The listing builds one solid part. Answer for the finished solid, in the listing's coordinates (mm). Round coordinates to 2 decimals unless told otherwise and drop trailing zeros. Write each loop counter-clockwise with the first axis right and the second up, starting at its lowest first coordinate (ties: lowest second). Pieces come first, ordered by that corner, then holes. Notation, with made-up numbers: M -2,88 L 36,88 A25 cw 36,123 Z; hole C 64,78.25 d3. An arc over 180 degrees is marked long. Answer as CSV lines item,"result". Start each with the question number.
from build123d import *

# Parameters (mm, degrees)
SKETCH22_R                       = 2.15
F_20_SERIES_TS20_40B_5MM_1_DEPTH = 225
M6X1_0_TAPPED_HOLE2_D            = 5
M6X1_0_TAPPED_HOLE2_DEPTH        = 15
M6X1_0_TAPPED_HOLE2_TIP          = 1.502151548


with BuildPart() as part:
    # Sketch22 → 20 series TS20-40B_5MM(1) (new body)
    with BuildSketch(Plane(origin=(0, 0, 0), x_dir=(-1, 0, 0), z_dir=(0, 1, 0))):
        with BuildLine():
            Line((-9.5, 7), (-8.476, 7))
            Line((-8.476, 7), (-8.476, 4.05))
            Line((-8.476, 4.05), (-7.063551759, 4.05))
            Line((-7.063551759, 4.05), (-4.5, 6.613551759))
            Line((-4.5, 6.613551759), (-4.5, 13.386448241))
            Line((-4.5, 13.386448241), (-7.063551759, 15.95))
            Line((-7.063551759, 15.95), (-8.476, 15.95))
            Line((-8.476, 15.95), (-8.476, 13))
            Line((-8.476, 13), (-9.5, 13))
            Line((-9.5, 13), (-9.5, 13.5))
            Line((-9.5, 13.5), (-10, 13.5))
            Line((-10, 13.5), (-10, 18.5014))
            ThreePointArc((-10, 18.5014), (-9.561070222, 19.561070222), (-8.5014, 20))
            Line((-8.5014, 20), (-3.5, 20))
            Line((-3.5, 20), (-3.5, 19.5))
            Line((-3.5, 19.5), (-3, 19.5))
            Line((-3, 19.5), (-3, 18.476))
            Line((-3, 18.476), (-5.95, 18.476))
            Line((-5.95, 18.476), (-5.95, 17.063551759))
            Line((-5.95, 17.063551759), (-3.386448241, 14.5))
            Line((-3.386448241, 14.5), (3.386448241, 14.5))
            Line((3.386448241, 14.5), (5.95, 17.063551759))
            Line((5.95, 17.063551759), (5.95, 18.476))
            Line((5.95, 18.476), (3, 18.476))
            Line((3, 18.476), (3, 19.5))
            Line((3, 19.5), (3.5, 19.5))
            Line((3.5, 19.5), (3.5, 20))
            Line((3.5, 20), (8.5014, 20))
            ThreePointArc((8.5014, 20), (9.561070222, 19.561070222), (10, 18.5014))
            Line((10, 18.5014), (10, 13.5))
            Line((10, 13.5), (9.5, 13.5))
            Line((9.5, 13.5), (9.5, 13))
            Line((9.5, 13), (8.476, 13))
            Line((8.476, 13), (8.476, 15.95))
            Line((8.476, 15.95), (7.063551759, 15.95))
            Line((7.063551759, 15.95), (4.5, 13.386448241))
            Line((4.5, 13.386448241), (4.5, 6.613551759))
            Line((4.5, 6.613551759), (7.063551759, 4.05))
            Line((7.063551759, 4.05), (8.476, 4.05))
            Line((8.476, 4.05), (8.476, 7))
            Line((8.476, 7), (9.5, 7))
            Line((9.5, 7), (9.5, 6.5))
            Line((9.5, 6.5), (10, 6.5))
            Line((10, 6.5), (10, -6.5))
            Line((10, -6.5), (9.5, -6.5))
            Line((9.5, -6.5), (9.5, -7))
            Line((9.5, -7), (8.476, -7))
            Line((8.476, -7), (8.476, -4.05))
            Line((8.476, -4.05), (7.063551759, -4.05))
            Line((7.063551759, -4.05), (4.5, -6.613551759))
            Line((4.5, -6.613551759), (4.5, -13.386448241))
            Line((4.5, -13.386448241), (7.063551759, -15.95))
            Line((7.063551759, -15.95), (8.476, -15.95))
            Line((8.476, -15.95), (8.476, -13))
            Line((8.476, -13), (9.5, -13))
            Line((9.5, -13), (9.5, -13.5))
            Line((9.5, -13.5), (10, -13.5))
            Line((10, -13.5), (10, -18.5014))
            ThreePointArc((10, -18.5014), (9.561070222, -19.561070222), (8.5014, -20))
            Line((8.5014, -20), (3.5, -20))
            Line((3.5, -20), (3.5, -19.5))
            Line((3.5, -19.5), (3, -19.5))
            Line((3, -19.5), (3, -18.476))
            Line((3, -18.476), (5.95, -18.476))
            Line((5.95, -18.476), (5.95, -17.063551759))
            Line((5.95, -17.063551759), (3.386448241, -14.5))
            Line((3.386448241, -14.5), (-3.386448241, -14.5))
            Line((-3.386448241, -14.5), (-5.95, -17.063551759))
            Line((-5.95, -17.063551759), (-5.95, -18.476))
            Line((-5.95, -18.476), (-3, -18.476))
            Line((-3, -18.476), (-3, -19.5))
            Line((-3, -19.5), (-3.5, -19.5))
            Line((-3.5, -19.5), (-3.5, -20))
            Line((-3.5, -20), (-8.5014, -20))
            ThreePointArc((-8.5014, -20), (-9.561070222, -19.561070222), (-10, -18.5014))
            Line((-10, -18.5014), (-10, -13.5))
            Line((-10, -13.5), (-9.5, -13.5))
            Line((-9.5, -13.5), (-9.5, -13))
            Line((-9.5, -13), (-8.476, -13))
            Line((-8.476, -13), (-8.476, -15.95))
            Line((-8.476, -15.95), (-7.063551759, -15.95))
            Line((-7.063551759, -15.95), (-4.5, -13.386448241))
            Line((-4.5, -13.386448241), (-4.5, -6.613551759))
            Line((-4.5, -6.613551759), (-7.063551759, -4.05))
            Line((-7.063551759, -4.05), (-8.476, -4.05))
            Line((-8.476, -4.05), (-8.476, -7))
            Line((-8.476, -7), (-9.5, -7))
            Line((-9.5, -7), (-9.5, -6.5))
            Line((-9.5, -6.5), (-10, -6.5))
            Line((-10, -6.5), (-10, 6.5))
            Line((-10, 6.5), (-9.5, 6.5))
            Line((-9.5, 6.5), (-9.5, 7))
        make_face()
        with Locations((0, 10)):
            Circle(SKETCH22_R, mode=Mode.SUBTRACT)
        with Locations((0, -10)):
            Circle(SKETCH22_R, mode=Mode.SUBTRACT)
        Polygon((-3.45829029, 5.5), (-6.43229029, 2.526), (-8.476, 2.526), (-8.476, -2.526), (-6.43229029, -2.526), (-3.45829029, -5.5), (3.45829029, -5.5), (6.43229029, -2.526), (8.476, -2.526), (8.476, 2.526), (6.43229029, 2.526), (3.45829029, 5.5), align=None, mode=Mode.SUBTRACT)
    extrude(amount=F_20_SERIES_TS20_40B_5MM_1_DEPTH)

    # M6x1.0 Tapped Hole2
    with Locations(Plane(origin=(0, 0, 0), x_dir=(-1, 0, 0), z_dir=(0, -1, 0))):
        with Locations((0, 10), (0, -10)):
            Hole(M6X1_0_TAPPED_HOLE2_D / 2, depth=M6X1_0_TAPPED_HOLE2_DEPTH)
            with Locations((0, 0, -(M6X1_0_TAPPED_HOLE2_DEPTH + M6X1_0_TAPPED_HOLE2_TIP / 2))):  # 118° drill point
                Cone(0, M6X1_0_TAPPED_HOLE2_D / 2, M6X1_0_TAPPED_HOLE2_TIP, mode=Mode.SUBTRACT)


solid = part.part
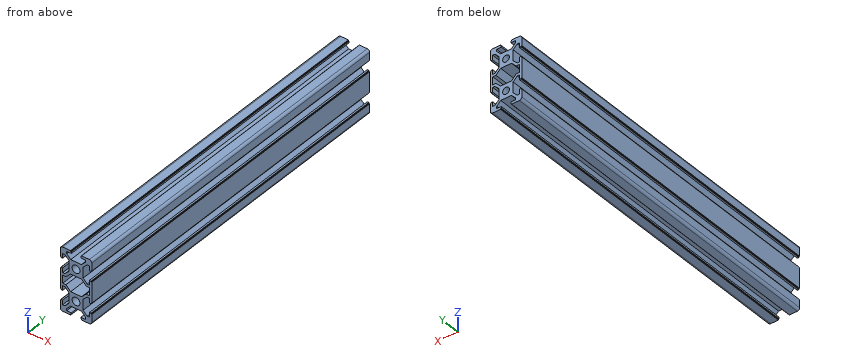
Q1. Straight lines are drawn through the part: L1, parallel to X at y = 84, z = 4.5; L2, parallel to Z at x = 0, y = 173; L3, parallel to Z at x = 0, y = 6. For each, find the intervals that lie inside material, in ascending order.
Q2. Find section B-B (x = 0). Determine the outline of the cut face in (y, z).
Q3. Find section A-A (z = -10). Determine the outline of the cut face in (x, y), plus the area to 3 significant figures.
Q4. Find section C-C (y = 202.5). Count the separate pieces of the cut face and the enclosed holes in it, plus the area to 3 significant figures.
Q5. Each of these flat-tipped pins is pushed along its axis until it touches: P1, Ø0.6, axis at y = 156.5, z = 19.5, coming from the -X side; P2, Ø0.5, axis at x = -9, y = 82, coming from the -Z side; P3, Ø0.6, axis at x = 10, y = 167, coming from the -Z side. Where does it stop, or does it pass through?
Reported:
1,L1,"x = -10 to -8.48, -6.61 to -4.46, 4.46 to 6.61, 8.48 to 10"
1,L2,"z = -14.5 to -12.15, -7.85 to -5.5, 5.5 to 7.85, 12.15 to 14.5"
1,L3,"z = -14.5 to -12.5, -7.5 to -5.5, 5.5 to 7.5, 12.5 to 14.5"
2,outline,"M 0,-14.5 L 225,-14.5 L 225,-12.15 L 15.21,-12.15 L 15,-12.5 L 0,-12.5 Z; M 0,-7.5 L 15,-7.5 L 15.21,-7.85 L 225,-7.85 L 225,-5.5 L 0,-5.5 Z; M 0,5.5 L 225,5.5 L 225,7.85 L 15.21,7.85 L 15,7.5 L 0,7.5 Z; M 0,12.5 L 15,12.5 L 15.21,12.15 L 225,12.15 L 225,14.5 L 0,14.5 Z"
3,outline,"M -4.5,0 L -2.5,0 L -2.5,15 L -2.15,15.21 L -2.15,225 L -4.5,225 Z; M 2.15,15.21 L 2.5,15 L 2.5,0 L 4.5,0 L 4.5,225 L 2.15,225 Z"
3,area,"1,050 mm2"
4,separate pieces,"1"
4,enclosed holes,"3"
4,area,"322 mm2"
5,P1,"stops at x = -9.83"
5,P2,"stops at z = -19.98"
5,P3,"stops at z = -19.4"
